```python
from build123d import *

# Parameters (mm, degrees)
SKETCH_2_R          = 35
EXTRUDE_1_DEPTH     = 42
FILLET_2_R          = 22
SKETCH_3_R          = 16
CUT_EXTRUDE_1_DEPTH = 20


with BuildPart() as part:
    # 草图1 → 旋转1 (revolve)
    with BuildSketch(Plane.XY, mode=Mode.PRIVATE) as revolve_1_sk:
        Polygon((0, 0), (0, 19), (22, 19), (22, 15), (32, 15), (32, 19), (57, 19), (57, 15), (112, 15), (112, 0), align=None)
    revolve(revolve_1_sk.sketch.rotate(Axis((0, 0, 0), (1, 0, 0)), 90), axis=Axis((0, 0, 0), (1, 0, 0)))

    # 草图2 → 凸台-拉伸1 (add, symmetric)
    with BuildSketch(Plane(origin=(0, 0, 0), x_dir=(1, 0, 0), z_dir=(0, 1, 0))):
        with Locations(Location((110, 0, 0), (0, 0, 270))):
            Circle(SKETCH_2_R)
    extrude(amount=EXTRUDE_1_DEPTH, both=True)

    # 圆角2
    fillet_2_edges = [part.edges().sort_by_distance(p)[0] for p in [
        (110, -42, -35),
        (110, 42, -35),
    ]]
    fillet(fillet_2_edges, radius=FILLET_2_R)

    # 草图3 → 切除-拉伸1 (cut)
    with BuildSketch(Plane.ZY):
        Circle(SKETCH_3_R)
    extrude(amount=-CUT_EXTRUDE_1_DEPTH, mode=Mode.SUBTRACT)


solid = part.part
```
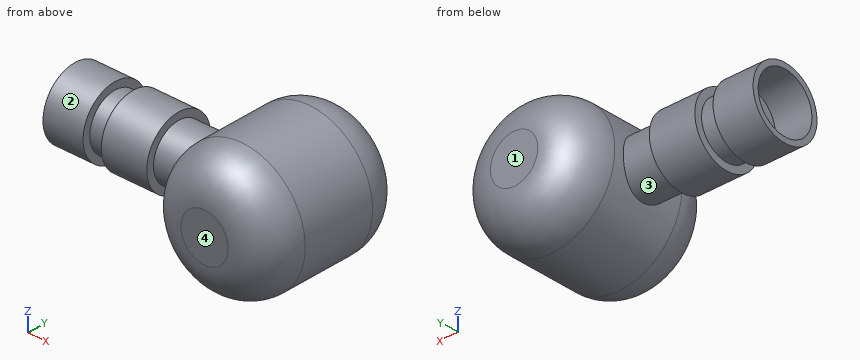
The listing builds one solid part. Answer for the finished solid, in the listing's coordinates (mm). Face numbers are marked on the shaded views. A direction names the side the tool comes from. Round coordinates to 2 decimals unless told otherwise and drop trailing zeros. Loops run counter-clockwise (first coordinate to the right, second up) from the corner with the lowest first, then second, coordinate; pieces in that order, holes last.
Q1. Section A-A, the plane y = 0 is taken. Determine the outline of the cut face in (x, z), then the cut area to 3 significant figures.
Q2. For a pull along X with two mould halves and no side action, classify the marked faces 3 and 4 as released by +X, released by -X, zero draft, split by the parting line, or undercut.
Q3. Section B-B, the plane x = 46 is taken. Determine the outline of the cut face in (y, z).
Q4. Find the intervals of material crossed by line 1 (Y direction, x = 7.75, z = 0); line 2 (Y direction, x = 61, z = 1); line 3 (X direction, y = -6, z = 16), in increasing order.
Q5. Section C-C, the plane y = 9 is taken. Determine the outline of the cut face in (x, z).
Q6. Given pin 1 Ø1.5 at (y, z) = (27, 1) entering from -X; pin 2 Ø3 at (y, z) = (4.5, -0.5) entering from +X; pin 3 Ø12 at (x, z) = (50.5, -20) entering from -Y, each flat-ended and moving along its own axis, determine where each tip first touches the part or whether it passes through.
Q7. Which of the six approach directions +Z, -Z, +X, -X, +Y, -Y give full straight-line access (tool end or side, diameter ignored) to the marked faces 1 and 2?
Completed:
1. outline: (0, -19) - (22, -19) - (22, -15) - (32, -15) - (32, -19) - (57, -19) - (57, -15) - (78.38, -15) arc R35 ccw (long way) to (78.38, 15) - (57, 15) - (57, 19) - (32, 19) - (32, 15) - (22, 15) - (22, 19) - (0, 19) - (0, 16) - (20, 16) - (20, -16) - (0, -16) - close
1. area: 5,870 mm2
2. face 3: undercut
2. face 4: zero draft
3. outline: circle Ø38 at (0, 0)
4. line 1: y = -19 to -16, 16 to 19
4. line 2: y = -14.97 to 14.97
4. line 3: x = 0 to 22, 32 to 57, 78.87 to 141.13
5. outline: (0, -16.73) - (22, -16.73) - (22, -12) - (32, -12) - (32, -16.73) - (57, -16.73) - (57, -12) - (77.12, -12) arc R35 ccw (long way) to (77.12, 12) - (57, 12) - (57, 16.73) - (32, 16.73) - (32, 12) - (22, 12) - (22, 16.73) - (0, 16.73) - (0, 13.23) - (20, 13.23) - (20, -13.23) - (0, -13.23) - close
6. pin 1: stops at x = 75.92
6. pin 2: stops at x = 145
6. pin 3: stops at y = -12.85
7. face 1: +Z, -Z, +X, -X, +Y
7. face 2: -X
